from build123d import *

# Parameters (mm, degrees)
SKETCH1_R           = 48.26
SKETCH1_R_2         = 27.051
BOSS_EXTRUDE1_DEPTH = 5.08
CUT_EXTRUDE1_DEPTH  = 69.438743413
SKETCH3_R           = 4.826
CUT_EXTRUDE2_DEPTH  = 69.29129044


with BuildPart() as part:
    # Sketch1 → Boss-Extrude1 (new body)
    with BuildSketch(Plane(origin=(0, 0, 0), x_dir=(1, 0, 0), z_dir=(0, 1, 0))):
        with Locations(Location((0, 0, 0), (0, 0, 270))):
            Circle(SKETCH1_R)
        with Locations(Location((0, 0, 0), (0, 0, 270))):
            Circle(SKETCH1_R_2, mode=Mode.SUBTRACT)
    extrude(amount=BOSS_EXTRUDE1_DEPTH)

    # Sketch2 → Cut-Extrude1 (cut, through all)
    with BuildSketch(Plane(origin=(0, 5.08, 0), x_dir=(1, 0, 0), z_dir=(0, 1, 0))):
        with BuildLine():
            ThreePointArc((-34.142692849, -3.175), (-34.29, 0), (-34.142692849, 3.175))
            Line((-34.142692849, 3.175), (-48.155445954, 3.175))
            ThreePointArc((-48.155445954, 3.175), (-48.26, 0), (-48.155445954, -3.175))
            Line((-48.155445954, -3.175), (-34.142692849, -3.175))
        make_face()
        with BuildLine():
            ThreePointArc((48.26, 0), (48.233854406, 1.588360519), (48.155445954, 3.175))
            Line((48.155445954, 3.175), (34.142692849, 3.175))
            ThreePointArc((34.142692849, 3.175), (34.29, 0), (34.142692849, -3.175))
            Line((34.142692849, -3.175), (48.155445954, -3.175))
            ThreePointArc((48.155445954, -3.175), (48.233854406, -1.588360519), (48.26, 0))
        make_face()
        with BuildLine():
            Line((-3.175, -34.142692849), (-3.175, -48.155445954))
            ThreePointArc((-3.175, -48.155445954), (0, -48.26), (3.175, -48.155445954))
            Line((3.175, -48.155445954), (3.175, -34.142692849))
            ThreePointArc((3.175, -34.142692849), (0, -34.29), (-3.175, -34.142692849))
        make_face()
        with BuildLine():
            ThreePointArc((3.175, 48.155445954), (0, 48.26), (-3.175, 48.155445954))
            Line((-3.175, 48.155445954), (-3.175, 34.142692849))
            ThreePointArc((-3.175, 34.142692849), (0, 34.29), (3.175, 34.142692849))
            Line((3.175, 34.142692849), (3.175, 48.155445954))
        make_face()
    extrude(amount=-CUT_EXTRUDE1_DEPTH, mode=Mode.SUBTRACT)

    # Sketch3 → Cut-Extrude2 (cut, through all)
    with BuildSketch(Plane(origin=(0, 5.08, 0), x_dir=(1, 0, 0), z_dir=(0, 1, 0))):
        with Locations(Location((-26.665276966, -26.665276966, 0), (0, 0, 270))):
            Circle(SKETCH3_R)
        with Locations(Location((26.626459399, 26.626459399, 0), (0, 0, 270))):
            Circle(SKETCH3_R)
    extrude(amount=-CUT_EXTRUDE2_DEPTH, mode=Mode.SUBTRACT)


solid = part.part
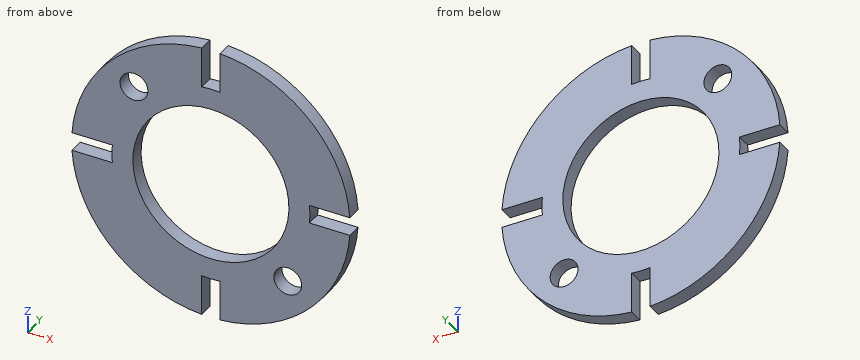
CAD build for the part. Positions are in the model's coordinates, mm. Round coordinates to 2 decimals unless told otherwise and drop trailing zeros. Write each loop counter-clockwise with the first axis right and the second up, starting at its lowest first coordinate (ties: lowest second). Pieces come first, ordered by that corner, then holes. Notation, with made-up numbers: (-23, 71) -> (-14, 71) arc R19 ccw to (-14, 78) -> close; hole circle Ø9 at (58.25, 27). An arc over 180 degrees is marked (long way). Answer as a JSON object with one key per item and string values.
(1) Band-saw the part on B-B, the plane z = 0. List the corners of the cut face in (x, y).
Reported:
{"outline": "(-34.29, 0) -> (-27.05, 0) -> (-27.05, 5.08) -> (-34.29, 5.08) -> close; (27.05, 0) -> (34.29, 0) -> (34.29, 5.08) -> (27.05, 5.08) -> close"}
(2) Probe probe 1 along X at (y, z) = (2.25, 0); probe 2 along X at (y, z) = (2.25, 25); probe 3 along X at (y, z) = (2.7, -23.5). List the from-to ranges inside material, lowest first. Write a range as [from, to].
Reported:
{"probe 1": "x = [-34.29, -27.05], [27.05, 34.29]", "probe 2": "x = [-41.28, -31.19], [-22.14, -10.33], [10.33, 41.28]", "probe 3": "x = [-42.15, -13.4], [13.4, 22.95], [30.3, 42.15]"}
(3) Pin check, flat tips, straight feed: P1, Ø3, axis at y = 3.5, z = -1, coming from the -X side; P2, Ø1.5, axis at x = 41.5, y = 3.5, coming from the +Z side; P3, Ø2.5, axis at x = 43, y = 1.5, coming from the -Z side. Stop position of each tip, or through.
Reported:
{"P1": "stops at x = -34.29", "P2": "stops at z = 25.85", "P3": "stops at z = -24.21"}
(4) Band-saw the part on C-C, the plane y = 2.75. List the corners of the cut face in (x, z) (3 decimals).
Reported:
{"outline": "(-48.155, -3.175) arc R48.26 ccw to (-3.175, -48.155) -> (-3.175, -34.143) arc R34.29 ccw to (3.175, -34.143) -> (3.175, -48.155) arc R48.26 ccw to (48.155, -3.175) -> (34.143, -3.175) arc R34.29 ccw to (34.143, 3.175) -> (48.155, 3.175) arc R48.26 ccw to (3.175, 48.155) -> (3.175, 34.143) arc R34.29 ccw to (-3.175, 34.143) -> (-3.175, 48.155) arc R48.26 ccw to (-48.155, 3.175) -> (-34.143, 3.175) arc R34.29 ccw to (-34.143, -3.175) -> close; hole circle Ø9.652 at (-26.665, 26.665); hole circle Ø54.102 at (0, 0); hole circle Ø9.652 at (26.626, -26.626)"}
(5) Band-saw the part on A-A, the plane x = 0. List the corners of the cut face in (y, z), then the cut area to 3 significant figures.
Reported:
{"outline": "(0, -34.29) -> (5.08, -34.29) -> (5.08, -27.05) -> (0, -27.05) -> close; (0, 27.05) -> (5.08, 27.05) -> (5.08, 34.29) -> (0, 34.29) -> close", "area": "73.5 mm^2"}
